from build123d import *

# Parameters (mm, degrees)
F0_W          = 2
F0_H          = 12
F1_DEPTH      = 48
F2_W          = 16
F2_H          = 7
F3_DEPTH      = 2.001
F3_DEPTH_BACK = 8
F4_R          = 2


with BuildPart() as f1:
    # F0 (on Right) → F1 (new body)
    with BuildSketch(Plane.YZ):
        Polygon((0, 2), (0, 0), (14, 0), (14, 2), (12, 2), align=None)
        with Locations((13, 8)):
            Rectangle(F0_W, F0_H)
    extrude(amount=F1_DEPTH)

    # F2 (on face) → F3 (cut, two sides)
    with BuildSketch(Plane.XZ.offset(-12)) as f3_sk:
        with Locations((24, 3.5)):
            Rectangle(F2_W, F2_H)
    extrude(amount=-F3_DEPTH, mode=Mode.SUBTRACT)
    extrude(f3_sk.sketch, amount=F3_DEPTH_BACK, mode=Mode.SUBTRACT)

    # F4
    f4_edges = [f1.edges().sort_by_distance(p)[0] for p in [
        (32, 4, 1),
        (16, 4, 1),
        (16, 13, 7),
        (32, 13, 7),
        (40, 12, 2),
        (8, 12, 2),
    ]]
    fillet(f4_edges, radius=F4_R)


solid = f1.part
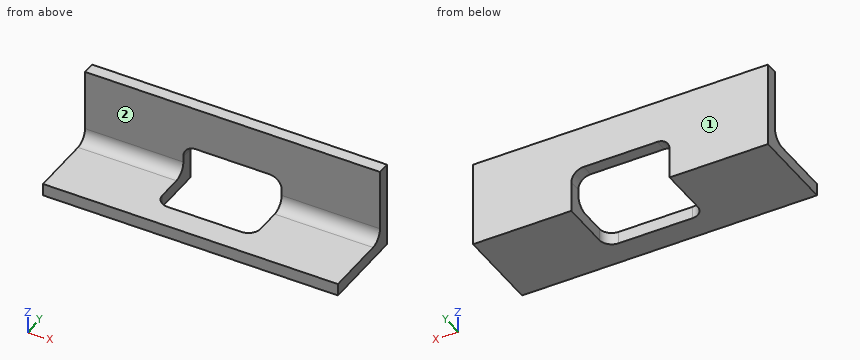
Could you check a few things on this model? Use its own coordinates, in mm. Face numbers are marked on the shaded views. A direction names the side the tool comes from. Give positions to 0.01 mm unless a question says otherwise; leave off trailing zeros. Order: outer loops, then holes, each group sorted by start corner. A loop starts at its lowest first (then second) coordinate and runs counter-clockwise, first axis right, second up. Notation, with made-up numbers: (-31, 61) -> (-18, 61) arc R28 cw to (-18, 88) -> close; hole circle Ø4 at (71.25, 9). An arc over 180 degrees is marked (long way). Answer in a Markdown table with one row per item. Add a question column.
Item 1: For the marked faces 1 and 2, which set-ups out of +Z, -Z, +X, -X, +Y, -Y let a thin tool reach every point of the face, with its end or its side?
Item 2: Imagine slicing it at A-A (y = 7.5). List the corners of the cut face in (x, z) for me, and give its area (3 significant figures).
Item 3: Imagine slicing it at D-D (z = 1.5). List the corners of the cut face in (x, y) for me, and give its area (3 significant figures).
Item 4: Imagine slicing it at B-B (x = 4). List the corners of the cut face in (y, z) for me.
Item 5: Please list where these lines run through material, in increasing order: probe 1 along X at (y, z) = (7.25, 1.25); probe 2 along Y at (x, z) = (46.5, 6.5); probe 3 along Z at (x, y) = (16, 3.25).
Item 6: I'm going to push flat-ended pins straight in: P1, Ø3, axis at x = 24, z = 11.5, coming from the -Y side; P2, Ø5, axis at x = 22, y = 6, coming from the +Z side; P3, Ø2, axis at x = 27, y = 12.5, coming from the -Z side. Where does each tip first touch, or does it pass through?
Item 7: Imagine slicing it at C-C (z = 6). List the corners of the cut face in (x, y) for me.
Result:
| question | item | result |
|---|---|---|
| 1 | face 1 | +Z, -Z, +X, -X, +Y |
| 1 | face 2 | +Z, +X, -X, -Y |
| 2 | outline | (0, 0) -> (16, 0) -> (16, 2) -> (0, 2) -> close; (32, 0) -> (48, 0) -> (48, 2) -> (32, 2) -> close |
| 2 | area | 64.0 mm2 |
| 3 | outline | (0, 0) -> (48, 0) -> (48, 14) -> (32, 14) -> (32, 6) arc R2 cw to (30, 4) -> (18, 4) arc R2 cw to (16, 6) -> (16, 14) -> (0, 14) -> close |
| 3 | area | 514 mm2 |
| 4 | outline | (0, 0) -> (14, 0) -> (14, 14) -> (12, 14) -> (12, 4) arc R2 cw to (10, 2) -> (0, 2) -> close |
| 5 | probe 1 | 0 to 16, 32 to 48 |
| 5 | probe 2 | 12 to 14 |
| 5 | probe 3 | 0 to 2 |
| 6 | P1 | y = 12 |
| 6 | P2 | z = 2 |
| 6 | P3 | z = 7 |
| 7 | outline | (0, 12) -> (16.27, 12) -> (16.27, 14) -> (0, 14) -> close; (31.73, 12) -> (48, 12) -> (48, 14) -> (31.73, 14) -> close |
